Read the model definition and answer for the solid it produces. Units are mm, in the model's axes. Face numbers are marked on the shaded views. Coordinates: 2 decimals unless noted, no trailing zeros. Write each loop counter-clockwise with the first axis right and the second up, starting at its lowest first coordinate (ties: lowest second). Pieces come first, ordered by that corner, then holes.
(1) Section A-A on x = 0 is taken. Write down the section's boundary in (y, z).
(2) Section D-D on y = 32 is taken. Write down the section's boundary in (x, z), then the cut area to 3 significant figures.
(3) Find the intervals of material crossed by probe 1 along Y at (x, z) = (3.5, -0.5); probe 2 along Y at (x, z) = (9, -7); probe 3 along Z at (x, y) = (-1, 21.5), in increasing order.
(4) Section C-C on y = 8 is taken. Write down the section's boundary in (x, z).
(5) The mould has two halves that part along Y. Classify the marked faces 1, 2 and 3: +Y half, -Y half, draft (parallel to the pull), parting line (faces both ways), or undercut.
(6) Section B-B on z = 0 is taken. Write down the section's boundary in (x, y), then the cut area to 3 significant figures.
(7) Given pin 1 (5 mm diameter, centred on x = 3, y = 31, fed in from -Z); pin 2 (2 mm diameter, centred on x = -8, z = 13, fed in from +Y), each flat-ended and moving along its own axis, determine where each tip first touches the part or whether it passes through.
from build123d import *

# Parameters (mm, degrees)
SKETCH1_R                = 17.5
BOSS_EXTRUDE1_DEPTH      = 6
CHAMFER1_SIZE            = 0.5
MOVE_START               = 6
MOVE_FACE1_OUTLINE_R     = 3.5
MOVE_FACE1_OUTLINE_R_2   = 2.5
MOVE_FACE1_DEPTH         = 3
MOVE_START_2             = 39
MOVE_FACE1_2_OUTLINE_R   = 2.5
MOVE_FACE1_2_OUTLINE_R_2 = 1.5
MOVE_FACE1_2_DEPTH       = 3.585600344
CHAMFER3_SIZE            = 0.5


# Read off the part's stored shape, not the designer's step: Move Face1
with BuildPart() as part:
    # Sketch1 → Boss-Extrude1 (new body)
    with BuildSketch(Plane(origin=(0, 0, 0), x_dir=(1, 0, 0), z_dir=(0, 1, 0))):
        with Locations(Location((0, 0, 0), (0, 0, 270))):
            Circle(SKETCH1_R)
    extrude(amount=BOSS_EXTRUDE1_DEPTH)

    # Chamfer1
    chamfer1_edges = [part.edges().sort_by_distance(p)[0] for p in [
        (0, 0, -17.5),
        (0, 6, -17.5),
    ]]
    chamfer(chamfer1_edges, length=CHAMFER1_SIZE)

    # Sketch3 → Revolve3 (revolve)
    with BuildSketch(Plane.XY, mode=Mode.PRIVATE) as revolve3_sk:
        with BuildLine():
            Line((-2.5, 6), (-2.5, 9))
            Line((-2.5, 9), (-5, 9))
            Line((-5, 9), (-5, 39))
            Line((-5, 39), (-1.5, 39))
            Line((-1.5, 39), (-1.5, 42))
            ThreePointArc((-1.5, 42), (-3.92634671, 46.472168293), (0, 49.708099244))
            Line((0, 49.708099244), (0, 6))
            Line((0, 6), (-2.5, 6))
        make_face()
    revolve(revolve3_sk.sketch.rotate(Axis((0, 0, 0), (0, 1, 0)), 270), axis=Axis((0, 0, 0), (0, 1, 0)))

    # Move Face1 outline → Move Face1 (add)
    with BuildSketch(Plane(origin=(0, 0, 0), x_dir=(1, 0, 0), z_dir=(0, 1, 0)).offset(MOVE_START)):
        Circle(MOVE_FACE1_OUTLINE_R)
        Circle(MOVE_FACE1_OUTLINE_R_2, mode=Mode.SUBTRACT)
    extrude(amount=MOVE_FACE1_DEPTH)

    # Move Face1 2 outline → Move Face1 2 (add)
    with BuildSketch(Plane(origin=(0, 0, 0), x_dir=(1, 0, 0), z_dir=(0, 1, 0)).offset(MOVE_START_2)):
        Circle(MOVE_FACE1_2_OUTLINE_R)
        Circle(MOVE_FACE1_2_OUTLINE_R_2, mode=Mode.SUBTRACT)
    extrude(amount=MOVE_FACE1_2_DEPTH)

    # Chamfer3
    chamfer3_edges = [part.edges().sort_by_distance(p)[0] for p in [
        (0, 39, 5),
        (0, 9, 5),
    ]]
    chamfer(chamfer3_edges, length=CHAMFER3_SIZE)


solid = part.part
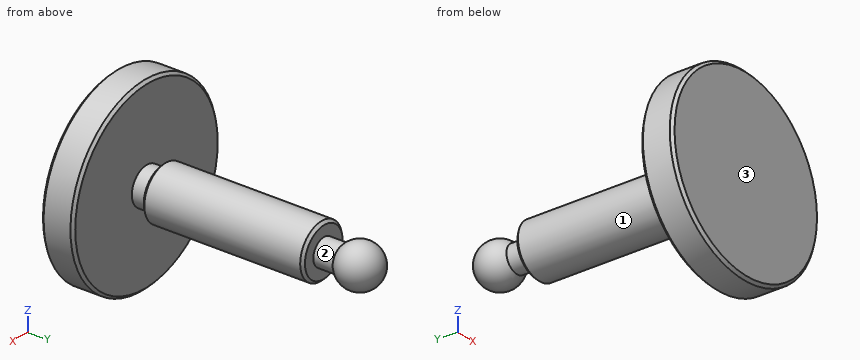
Response:
1. outline: (0, -17) - (0.5, -17.5) - (5.5, -17.5) - (6, -17) - (6, -3.5) - (9, -3.5) - (9, -4.5) - (9.5, -5) - (38.5, -5) - (39, -4.5) - (39, -2.5) - (42.59, -2.5) arc R4 ccw (long way) to (42.59, 2.5) - (39, 2.5) - (39, 4.5) - (38.5, 5) - (9.5, 5) - (9, 4.5) - (9, 3.5) - (6, 3.5) - (6, 17) - (5.5, 17.5) - (0.5, 17.5) - (0, 17) - close
2. outline: circle Ø10 at (0, 0)
2. area: 78.5 mm2
3. probe 1: y = 0 to 6, 9 to 39, 43.84 to 47.58
3. probe 2: y = 0 to 6
3. probe 3: z = -4.9 to 4.9
4. outline: circle Ø7 at (0, 0)
5. face 1: draft
5. face 2: undercut
5. face 3: -Y half
6. outline: (-17.5, 0.5) - (-17, 0) - (17, 0) - (17.5, 0.5) - (17.5, 5.5) - (17, 6) - (3.5, 6) - (3.5, 9) - (4.5, 9) - (5, 9.5) - (5, 38.5) - (4.5, 39) - (2.5, 39) - (2.5, 42.59) arc R4 ccw (long way) to (-2.5, 42.59) - (-2.5, 39) - (-4.5, 39) - (-5, 38.5) - (-5, 9.5) - (-4.5, 9) - (-3.5, 9) - (-3.5, 6) - (-17, 6) - (-17.5, 5.5) - close
6. area: 595 mm2
7. pin 1: stops at z = -4.97
7. pin 2: stops at y = 6
